Verification items for the finished model (mm, model axes). A direction names the side the tool comes from. Coordinates: 2 decimals unless noted, no trailing zeros. Write each loop counter-clockwise with the first axis right and the second up, starting at its lowest first coordinate (ties: lowest second). Pieces come first, ordered by that corner, then holes. Notation, with made-up numbers: (19, -29) -> (43, -29) arc R9 cw to (43, -25) -> close; hole circle Ø9 at (-26.5, 63). An arc over 180 degrees is marked (long way). Answer in a Markdown table with one row per item.
```python
from build123d import *

# Parameters (mm, degrees)
F0_W     = 609.6
F0_H     = 38.1
F0_R     = 6.35
F1_DEPTH = 152.4
F2_R     = 2.54
F4_DEPTH = 609.6


with BuildPart() as f1:
    # F0 (on Top) → F1 (new body)
    with BuildSketch(Plane.XY):
        with Locations((228.6, 0)):
            Rectangle(F0_W, F0_H)
        Circle(F0_R, mode=Mode.SUBTRACT)
        with Locations((152.4, 0)):
            Circle(F0_R, mode=Mode.SUBTRACT)
        with Locations((304.8, 0)):
            Circle(F0_R, mode=Mode.SUBTRACT)
        with Locations((457.2, 0)):
            Circle(F0_R, mode=Mode.SUBTRACT)
    extrude(amount=-F1_DEPTH)

    # F2
    f2_edges = [f1.edges().sort_by_distance(p)[0] for p in [
        (228.6, 19.05, 0),
        (228.6, 19.05, -152.4),
    ]]
    fillet(f2_edges, radius=F2_R)

    # F3 (on face) → F4 (cut, through all)
    with BuildSketch(Plane(origin=(-76.2, 0, 0), x_dir=(0, -1, 0), z_dir=(-1, 0, 0))):
        with BuildLine():
            Line((-16.51, -150.282402), (19.05, -150.282402))
            Line((19.05, -150.282402), (19.05, -2.117598))
            Line((19.05, -2.117598), (-16.51, -2.117598))
            ThreePointArc((-16.51, -2.117598), (-16.808684, -2.241316), (-16.932402, -2.54))
            Line((-16.932402, -2.54), (-16.932402, -149.86))
            ThreePointArc((-16.932402, -149.86), (-16.808684, -150.158684), (-16.51, -150.282402))
        make_face()
    extrude(amount=-F4_DEPTH, mode=Mode.SUBTRACT)


solid = f1.part
```
1. Tool access check on faces 1 (the cylindrical face through (463.066, -2.432, -1.044)), 2 (the flat face through (224, -2, -2.118)). Record the directions out of +Z, -Z, +X, -X, +Y, -Y that give a thin tool (end or side, any length) a straight path to the whole face; none if there is none.
Geometry says:
| item | result |
|---|---|
| face 1 | +Z, -Z |
| face 2 | +X, -X, -Y |
2. Thickness scan on line 1 (Z direction, x = 299, y = 13); line 2 (Y direction, x = 367, z = -35.5); line 3 (Y direction, x = 0, z = -0.4). Record the ranges inside material, lowest first. Write a range as from..to.
Geometry says:
| item | result |
|---|---|
| line 1 | -152.4..-150.28, -2.12..0 |
| line 2 | 16.93..19.05 |
| line 3 | -19.05..-6.35, 6.35..17.88 |
3. Mould release check, pull along X, two halves, no side actions. Record for faces 3 (the flat face through (-76.2, 18, -76)), 4 (the flat face through (224, -1, -150.282)), 5 (the cylindrical face through (310.666, -2.432, -1.044)), 6 (the flat face through (533.4, 18, -76)): released by +X, released by -X, zero draft, split by the parting line, or undercut.
Geometry says:
| item | result |
|---|---|
| face 3 | released by -X |
| face 4 | zero draft |
| face 5 | undercut |
| face 6 | released by +X |
4. Section check A-A, the plane x = 152.4. Record the boundary of the cut face in (y, z), plus the area to 3 significant figures.
Geometry says:
| item | result |
|---|---|
| outline | (-19.05, -152.4) -> (-6.35, -152.4) -> (-6.35, -150.28) -> (-19.05, -150.28) -> close; (-19.05, -2.12) -> (-6.35, -2.12) -> (-6.35, 0) -> (-19.05, 0) -> close; (6.35, -152.4) -> (16.51, -152.4) arc R2.54 ccw to (19.05, -149.86) -> (19.05, -2.54) arc R2.54 ccw to (16.51, 0) -> (6.35, 0) -> (6.35, -2.12) -> (16.51, -2.12) arc R0.42 cw to (16.93, -2.54) -> (16.93, -149.86) arc R0.42 cw to (16.51, -150.28) -> (6.35, -150.28) -> close |
| area | 419 mm^2 |
5. Section check D-D, the plane x = 457.5. Record the boundary of the cut face in (y, z), plus the area to 3 significant figures.
Geometry says:
| item | result |
|---|---|
| outline | (-19.05, -152.4) -> (-6.34, -152.4) -> (-6.34, -150.28) -> (-19.05, -150.28) -> close; (-19.05, -2.12) -> (-6.34, -2.12) -> (-6.34, 0) -> (-19.05, 0) -> close; (6.34, -152.4) -> (16.51, -152.4) arc R2.54 ccw to (19.05, -149.86) -> (19.05, -2.54) arc R2.54 ccw to (16.51, 0) -> (6.34, 0) -> (6.34, -2.12) -> (16.51, -2.12) arc R0.42 cw to (16.93, -2.54) -> (16.93, -149.86) arc R0.42 cw to (16.51, -150.28) -> (6.34, -150.28) -> close |
| area | 419 mm^2 |
6. Section check C-C, the plane y = 0. State how many separate pieces and enclosed holes the cut face has, plus the area to 3 significant figures.
Geometry says:
| item | result |
|---|---|
| separate pieces | 10 |
| enclosed holes | 0 |
| area | 2,370 mm^2 |
7. Depth check by flat-ended pin: P1, Ø5, axis at x = 349.5, z = -56.5, coming from the -Y side. Enter the tip coordinate at first touch or a pass-through.
Geometry says:
| item | result |
|---|---|
| P1 | y = 16.93 |
8. Section check B-B, the plane x = 243. Record the boundary of the cut face in (y, z), plus the area to 3 significant figures.
Geometry says:
| item | result |
|---|---|
| outline | (-19.05, -152.4) -> (16.51, -152.4) arc R2.54 ccw to (19.05, -149.86) -> (19.05, -2.54) arc R2.54 ccw to (16.51, 0) -> (-19.05, 0) -> (-19.05, -2.12) -> (16.51, -2.12) arc R0.42 cw to (16.93, -2.54) -> (16.93, -149.86) arc R0.42 cw to (16.51, -150.28) -> (-19.05, -150.28) -> close |
| area | 472 mm^2 |
